For this review, take the finished solid that the model builds, in its own axes (mm). Face numbers are marked on the shaded views. A direction names the side the tool comes from. Round coordinates to 2 decimals unless told otherwise and drop trailing zeros. Order: outer loops, then holes, each group sorted by start corner. A loop starts at its lowest first (then second) coordinate and runs counter-clockwise, first axis right, second up. Notation, with made-up numbers: (56, 43.5) - (104, 43.5) arc R10 ccw to (104, 54.5) - close; hole circle Ø1 at (71, 52). An arc over 180 degrees is marked (long way). One line per question, with ' | ' between items.
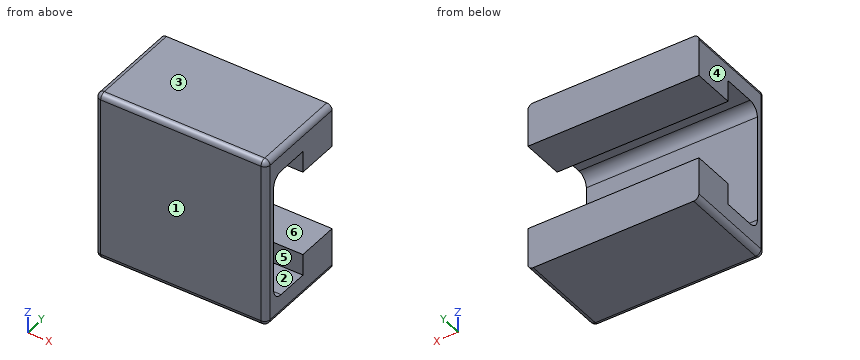
```python
from build123d import *

# Parameters (mm, degrees)
EXTRUDE_1_DEPTH = 8
FILLET_1_R      = 0.25


with BuildPart() as part:
    # 草圖1 → 填料-伸長1 (new body)
    with BuildSketch(Plane(origin=(0, 0, 0), x_dir=(0, 0, -1), z_dir=(1, 0, 0))):
        with BuildLine():
            Line((0, 0), (0, 4.5))
            Line((0, 4.5), (2, 4.5))
            Line((2, 4.5), (2, 2.5))
            Line((2, 2.5), (1, 2.5))
            Line((1, 2.5), (1, 1))
            ThreePointArc((1, 1), (1.146446609, 0.646446609), (1.5, 0.5))
            Line((1.5, 0.5), (6.5, 0.5))
            ThreePointArc((6.5, 0.5), (6.853553391, 0.646446609), (7, 1))
            Line((7, 1), (7, 2.5))
            Line((7, 2.5), (6, 2.5))
            Line((6, 2.5), (6, 4.5))
            Line((6, 4.5), (8, 4.5))
            Line((8, 4.5), (8, 0))
            Line((8, 0), (0, 0))
        make_face()
    extrude(amount=-EXTRUDE_1_DEPTH)

    # 圓角1
    fillet_1_edges = [part.edges().sort_by_distance(p)[0] for p in [
        (0, 2.25, 0),
        (0, 2.25, -8),
        (0, 0, -4),
        (-4, 0, 0),
        (-4, 0, -8),
        (-8, 0, -4),
        (-8, 2.25, 0),
        (-8, 2.25, -8),
    ]]
    fillet(fillet_1_edges, radius=FILLET_1_R)


solid = part.part
```
(1) We need section C-C on y = 1.2. State the section outline as (x, z) points, plus the area to 3 significant figures.
Output values:
outline: (-8, -7.75) arc R0.25 ccw to (-7.75, -8) - (-0.25, -8) arc R0.25 ccw to (0, -7.75) - (0, -7) - (-8, -7) - close; (-8, -1) - (0, -1) - (0, -0.25) arc R0.25 ccw to (-0.25, 0) - (-7.75, 0) arc R0.25 ccw to (-8, -0.25) - close | area: 15.9 mm^2
(2) For the marked faces 4, 5 and 6, list the 3-axis set-ups (+Z, -Z, +X, -X, +Y, -Y) from which the entire face can be reached by the end or side of a thin tool; tool diameter is ignored.
Output values:
face 4: +Z, -Z, -X, +Y, -Y | face 5: +X, -X | face 6: +X, -X, +Y
(3) We need section A-A on y = 4.1. State the section outline as (x, z) points, plus the area to 3 significant figures.
Output values:
outline: (-8, -7.75) arc R0.25 ccw to (-7.75, -8) - (-0.25, -8) arc R0.25 ccw to (0, -7.75) - (0, -6) - (-8, -6) - close; (-8, -2) - (0, -2) - (0, -0.25) arc R0.25 ccw to (-0.25, 0) - (-7.75, 0) arc R0.25 ccw to (-8, -0.25) - close | area: 31.9 mm^2
(4) For probe 1 along Z at (x, y) = (-6, 1.45); probe 2 along Y at (x, z) = (-5.25, -1.5); probe 3 along Z at (x, y) = (-2, 2.7), list the stretches that pass through material, from the lowest coordinate up. Write a range as [from, to].
Output values:
probe 1: [-8, -7], [-1, 0] | probe 2: [0, 0.5], [2.5, 4.5] | probe 3: [-8, -6], [-2, 0]
(5) We need section D-D on z = -5.5. State the section outline as (x, y) points, plus the area to 3 significant figures.
Output values:
outline: (-8, 0.25) arc R0.25 ccw to (-7.75, 0) - (-0.25, 0) arc R0.25 ccw to (0, 0.25) - (0, 0.5) - (-8, 0.5) - close | area: 3.97 mm^2
(6) Insertion check: pin 1 (1.5 mm diameter, centred on y = 3.5, z = -5.5, fed in from +X). The pin has a flat end and moves straight along its axis. Give the tip position at first contact, or say it passes through.
Output values:
pin 1: x = 0
(7) Mouldability with a two-part tool opening along Y and no side actions: class the marked faces 1, 2 and 3 as released by +Y, released by -Y, zero draft, split by the parting line, or undercut.
Output values:
face 1: released by -Y | face 2: undercut | face 3: zero draft
(8) We need section B-B on x = -4. State the section outline as (y, z) points.
Output values:
outline: (0, -7.75) arc R0.25 ccw to (0.25, -8) - (4.5, -8) - (4.5, -6) - (2.5, -6) - (2.5, -7) - (1, -7) arc R0.5 cw to (0.5, -6.5) - (0.5, -1.5) arc R0.5 cw to (1, -1) - (2.5, -1) - (2.5, -2) - (4.5, -2) - (4.5, 0) - (0.25, 0) arc R0.25 ccw to (0, -0.25) - close
